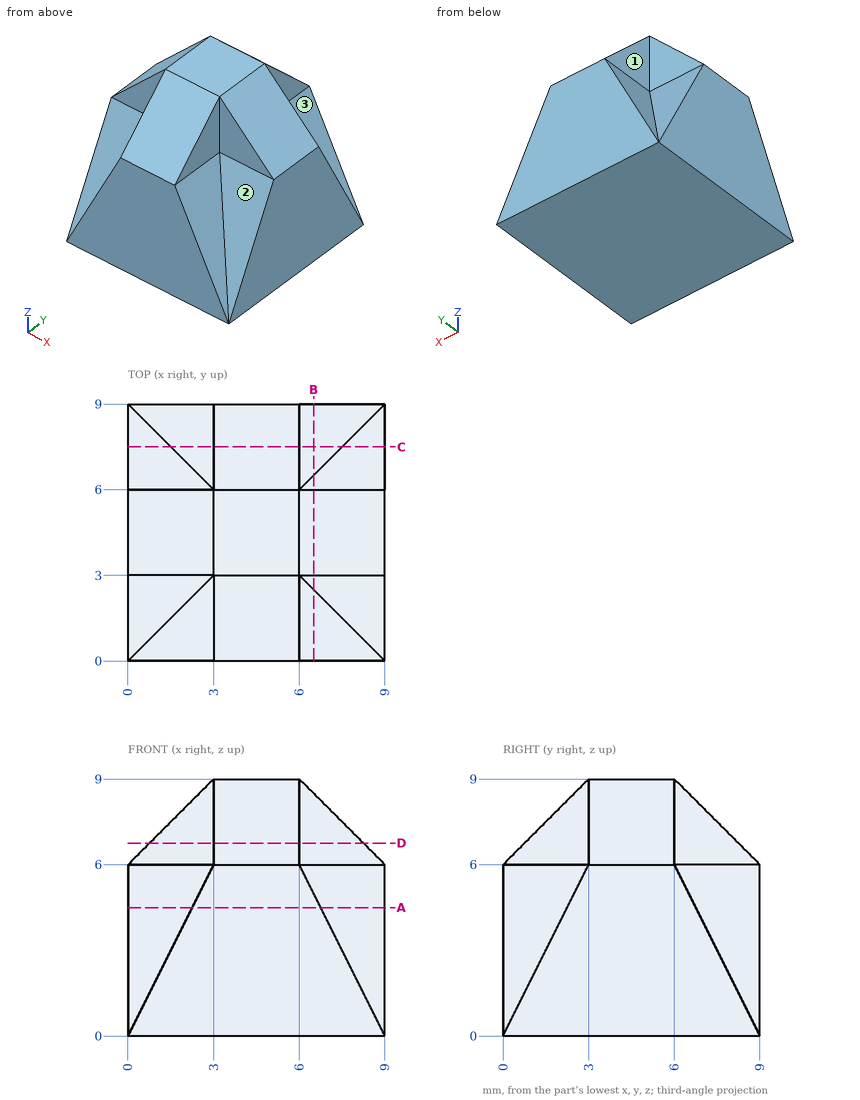
Geometry: see drawing. Coordinates: mm, zero at the bounding-box minimum. A direction names the side the tool comes from. Round coordinates to 2 decimals unless told otherwise and drop trailing zeros. Loops run counter-clockwise (first coordinate to the right, second up) from the corner with the lowest first, then second, coordinate; pieces in that order, holes last. Notation, with made-up numbers: M -5,65 L 11,65 A12 ccw 11,83 Z; hole C 54,63.25 d9. An arc over 180 degrees is marked long. Use a Markdown table: item, result. Add a question column.
1. Set-up query: the marked faces 1, 2 and 3. Return all of +Z, -Z, +X, -X, +Y, -Y with unobstructed straight access to the full face (end or side cutting, diameter ignored); none if empty.
2. Cut plane C-C, the plane y = 7.5. Output: boundary loops of the cut face in (x, z), and give its area (3 significant figures).
3. Contact query for flat-ended pins moving along their axis: pin 1 (0.9 mm diameter, centred on x = 1.5, z = 7, fed in from +Y); pin 2 (1.5 mm diameter, centred on x = 2, z = 8, fed in from -Y); pin 3 (1.5 mm diameter, centred on y = 1, z = 8, fed in from -X). Output: stop coordinate, or through.
4. Cut plane D-D, the plane z = 6.75. Output: boundary loops of the cut face in (x, y), and give its area (3 significant figures).
5. Cut plane A-A, the plane z = 4.5. Output: boundary loops of the cut face in (x, y), and give its area (4 significant figures).
6. Cut plane B-B, the plane x = 6.5. Output: boundary loops of the cut face in (y, z), and give its area (3 significant figures).
7. Ray query, line 1 along X through (y, z) = (6.75, 6.75); line 2 along Z through (x, y) = (1, 2.5); line 3 along Z through (x, y) = (7.75, 1). Return the intervals inside material, ascending. Write a range as [from, to].
Solution:
| question | item | result |
|---|---|---|
| 1 | face 1 | +Z, -X, +Y |
| 1 | face 2 | +Z, +X, -Y |
| 1 | face 3 | +Z, +X, +Y |
| 2 | outline | M 0,0 L 9,0 L 9,3 L 7.5,3 L 6,6 L 6,7.5 L 3,7.5 L 3,6 L 1.5,3 L 0,3 Z |
| 2 | area | 45.0 mm2 |
| 3 | pin 1 | stops at y = 6 |
| 3 | pin 2 | stops at y = 3 |
| 3 | pin 3 | stops at x = 3 |
| 4 | outline | M 0.75,3 L 3,3 L 3,0.75 L 6,0.75 L 6,3 L 8.25,3 L 8.25,6 L 6,6 L 6,8.25 L 3,8.25 L 3,6 L 0.75,6 Z |
| 4 | area | 36.0 mm2 |
| 5 | outline | M 0,2.25 L 2.25,2.25 L 2.25,0 L 6.75,0 L 6.75,2.25 L 9,2.25 L 9,6.75 L 6.75,6.75 L 6.75,9 L 2.25,9 L 2.25,6.75 L 0,6.75 Z |
| 5 | area | 60.75 mm2 |
| 6 | outline | M 0,0 L 9,0 L 9,5 L 6.5,5 L 6,6 L 6,8.5 L 3,8.5 L 3,6 L 2.5,5 L 0,5 Z |
| 6 | area | 56.0 mm2 |
| 7 | line 1 | x = [3, 6] |
| 7 | line 2 | z = [0, 5] |
| 7 | line 3 | z = [0, 2.5] |
